Verification items for the finished model (mm, model axes). A direction names the side the tool comes from. Give positions to 0.01 mm unless a question says otherwise; leave off trailing zeros. Order: outer loops, then holes, each group sorted by start corner. A loop starts at its lowest first (then second) coordinate and runs counter-clockwise, first axis right, second up. Notation, with made-up numbers: (61, 7) - (100, 7) arc R20 ccw to (100, 33) - close; hole circle Ø9 at (80.5, 41). An arc over 180 degrees is marked (long way). Answer as a JSON object with one key per item and string values. Group by question number.
(1) Thickness scan on line 1 (Y direction, x = 27, z = 13); line 2 (X direction, y = -8, z = 10.5). Record the ranges inside material, lowest first.
(2) Access from +Z, -Z, +X, -X, +Y, -Y to the whole of each face (thin tool, end or side, straight path). Record for faces 1 (the face through (68.605, 4.93, 26.299)), 2 (the face through (0, -19, 21)), 3 (the face through (-5, -11, 31)).
(3) Mould release check, pull along Z, two halves, no side actions. Record for faces 4 (the face through (64.22, 4.93, 22.13)), 5 (the face through (36, -15, 10)), 6 (the face through (71, -3, 8)), 7 (the face through (31, -9, 0)): +Z half, -Z half, draft (parallel to the pull), parting line (faces both ways), or undercut.
(4) Section check D-D (z = 18.5). Record the boundary of the cut face in (x, y), then the cut area to 3 significant figures.
(5) Section check B-B (z = 7). Record the boundary of the cut face in (x, y), then the cut area to 3 significant figures.
(6) Section check A-A (y = 2). Record the boundary of the cut face in (x, z).
(7) Section check C-C (x = 60). Record the boundary of the cut face in (y, z), then the cut area to 3 significant figures.
(8) Depth check by flat-ended pin: pin 1 Ø8 at (x, y) = (-3, -8) entering from +Z; pin 2 Ø19.5 at (x, y) = (49, -12) entering from +Z; pin 3 Ø8 at (x, z) = (45.5, 13) entering from -Y. Enter the tip coordinate at first touch or a pass-through.
```python
from build123d import *

# Parameters (mm, degrees)
BOSS_EXTRUDE1_DEPTH = 10
BOSS_EXTRUDE2_DEPTH = 10
SKETCH6_R           = 11
SKETCH6_R_2         = 5
BOSS_EXTRUDE3_DEPTH = 10


with BuildPart() as part:
    # Sketch1 → Boss-Extrude1 (new body)
    with BuildSketch(Plane.XY):
        Polygon((0, 0), (71, 0), (71, -22.60835843), (0, -39), align=None)
    extrude(amount=BOSS_EXTRUDE1_DEPTH)

    # Sketch3 → Boss-Extrude2 (add)
    with BuildSketch(Plane.ZY):
        Polygon((0, 0), (31, 0), (31, -23), (23, -39), (0, -39), align=None)
    extrude(amount=BOSS_EXTRUDE2_DEPTH)

    # Sketch6 → Boss-Extrude3 (add)
    # profile 1 of 2: a face of its own
    with BuildSketch(Plane(origin=(0, 0, 0), x_dir=(1, 0, 0), z_dir=(0, 1, 0))):
        with Locations((60, -19.446177938)):
            Circle(SKETCH6_R)
        with Locations(Location((60, -19.446177938, 0), (0, 0, 270))):
            Circle(SKETCH6_R_2, mode=Mode.SUBTRACT)
    # profile 2 of 2: a face of its own
    with BuildSketch(Plane(origin=(0, 0, 0), x_dir=(1, 0, 0), z_dir=(0, 1, 0))):
        with BuildLine():
            Line((71, -19.446177938), (71, 0))
            Line((71, 0), (-10, 0))
            Line((-10, 0), (-10, -43))
            Line((-10, -43), (11, -43))
            Line((11, -43), (62.661140852, -30.119430927))
            ThreePointArc((62.661140852, -30.119430927), (51.33188171, -12.673901709), (71, -19.446177938))
        make_face()
    extrude(amount=BOSS_EXTRUDE3_DEPTH)


solid = part.part
```
Solutions:
{
 "1": {"line 1": "y = 0 to 10", "line 2": "x = -10 to 0"},
 "2": {"face 1": "+Z, +X, +Y, -Y", "face 2": "+Z, +X, -Y", "face 3": "+Z, +X, -X, -Y"},
 "3": {"face 4": "undercut", "face 5": "+Z half", "face 6": "draft", "face 7": "-Z half"},
 "4": {"outline": "(-10, -39) - (0, -39) - (0, 0) - (55.09, 0) - (55.09, 10) - (-10, 10) - close; (64.91, 0) - (71, 0) - (71, 10) - (64.91, 10) - close", "area": "1,100 mm2"},
 "5": {"outline": "(-10, -39) - (0, -39) - (71, -22.61) - (71, 10) - (-10, 10) - close", "area": "3,390 mm2"},
 "6": {"outline": "(-10, 0) - (71, 0) - (71, 19.45) arc R11 ccw to (62.66, 30.12) - (11, 43) - (-10, 43) - close; hole circle Ø10 at (60, 19.45)"},
 "7": {"outline": "(-25.15, 0) - (10, 0) - (10, 14.45) - (0, 14.45) - (0, 10) - (-25.15, 10) - close; (0, 24.45) - (10, 24.45) - (10, 30.78) - (0, 30.78) - close", "area": "459 mm2"},
 "8": {"pin 1": "stops at z = 31", "pin 2": "stops at z = 10", "pin 3": "stops at y = -29.11"}
}
